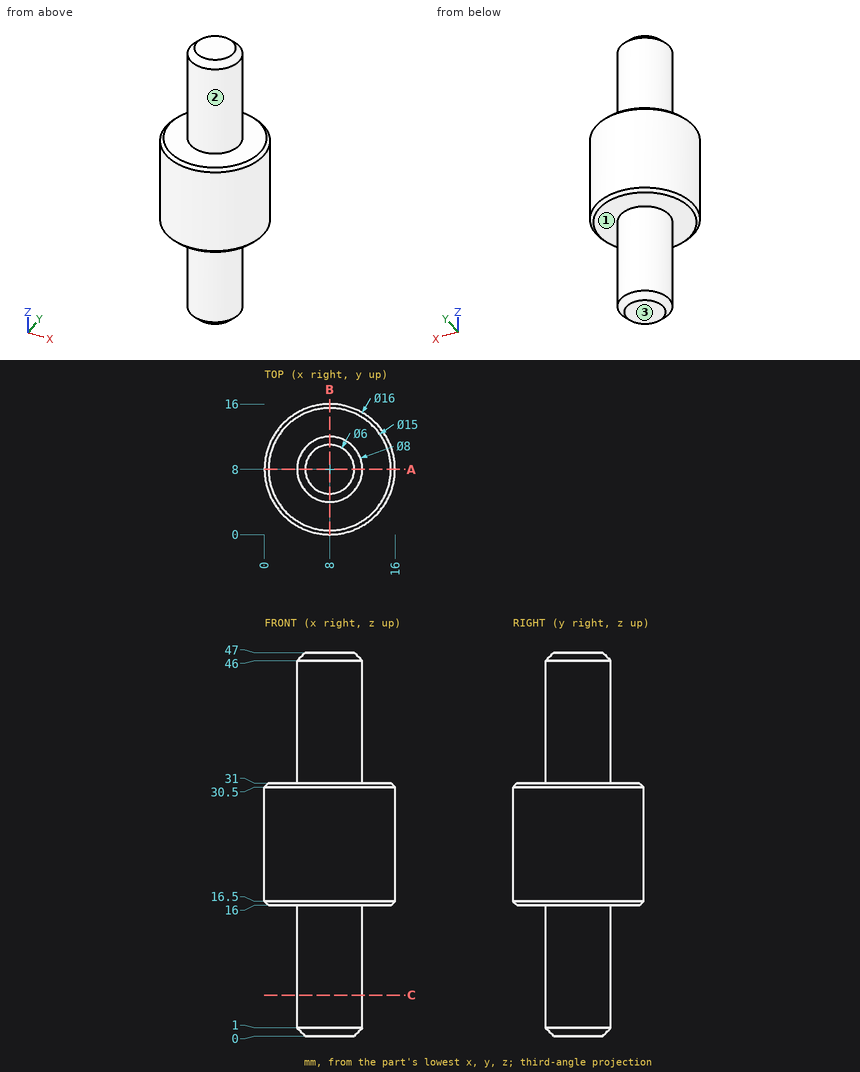
Answer from the drawing. Dimensions are ordinates in mm from the lowest x, y and z of the part. A direction names the side the tool comes from. Round coordinates to 2 decimals unless told otherwise and drop trailing zeros. Write each loop counter-clockwise with the first axis right and the second up, starting at its lowest first coordinate (ties: lowest second). Pieces come first, ordered by that corner, then holes.
1. Which of the six approach directions +Z, -Z, +X, -X, +Y, -Y give full straight-line access (tool end or side, diameter ignored) to the marked faces 1, 2 and 3?
2. Given pin 1 Ø4 at (x, y) = (4, 3) entering from -Z; pin 2 Ø4 at (y, z) = (4, 5.5) entering from -X; pin 3 Ø5 at (x, y) = (12, 2) entering from +Z; pin 4 Ø4.5 at (x, y) = (5, 8.5) entering from +Z, each flat-ended and moving along its own axis, determine where each tip first touches the part or whether it passes through.
3. Straight lines are drawn through the part: L1, parallel to Z at x = 3.5, y = 6.5; L2, parallel to Y at x = 13.5, z = 24; L3, parallel to X at y = 11, z = 39. For each, find the intervals that lie inside material, in ascending order.
4. The part is cut by section A-A, the plane y = 8. Determine the outline of the cut face in (x, z), then the cut area to 4 significant figures.
5. The part is cut by section C-C, the plane z = 5. Determine the outline of the cut face in (x, y).
Values:
1. face 1: -Z
1. face 2: +Z
1. face 3: -Z, +X, -X, +Y, -Y
2. pin 1: stops at z = 16
2. pin 2: stops at x = 4.54
2. pin 3: stops at z = 31
2. pin 4: stops at z = 47
3. L1: z = 16 to 31
3. L2: y = 2.19 to 13.81
3. L3: x = 5.35 to 10.65
4. outline: (0, 16.5) - (0.5, 16) - (4, 16) - (4, 1) - (5, 0) - (11, 0) - (12, 1) - (12, 16) - (15.5, 16) - (16, 16.5) - (16, 30.5) - (15.5, 31) - (12, 31) - (12, 46) - (11, 47) - (5, 47) - (4, 46) - (4, 31) - (0.5, 31) - (0, 30.5) - close
4. area: 493.5 mm2
5. outline: circle Ø8 at (8, 8)
